Geometry check sheet. Reference: drawing and pictorial views, mm from the part's lowest x, y, z. Give positions to 0.01 mm unless a question says otherwise; leave off trailing zeros. Order: outer loops, then holes, each group sorted by start corner. A loop starts at its lowest first (then second) coordinate and runs counter-clockwise, first axis right, second up.
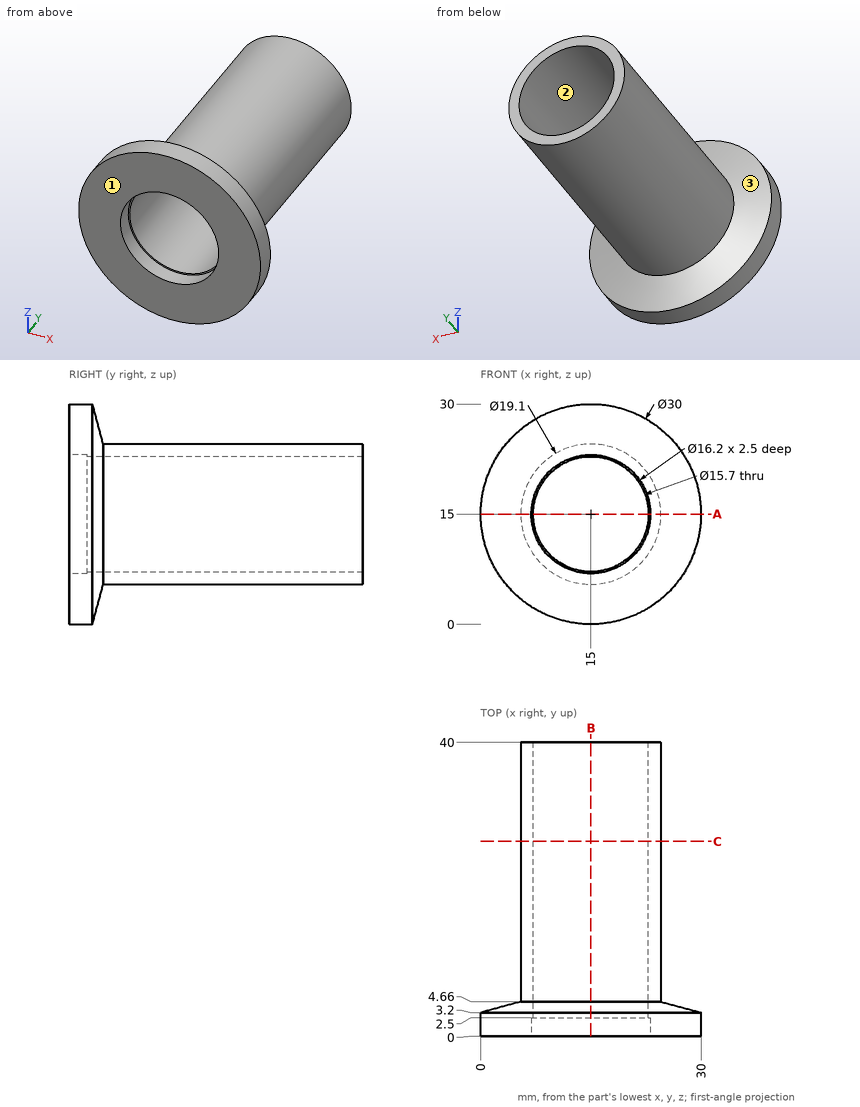
1) Draft check along Z on the marked faces 1, 2 and 3. Enter one of: +Z half, -Z half, draft (parallel to the pull), parting line (faces both ways), or undercut.
Recorded:
face 1: draft
face 2: undercut
face 3: parting line
2) Section check B-B, the plane x = 15. Record the cut outline in (y, z).
Recorded:
outline: (0, 0) - (3.2, 0) - (4.66, 5.45) - (40, 5.45) - (40, 7.15) - (2.5, 7.15) - (2.5, 6.9) - (0, 6.9) - close; (0, 23.1) - (2.5, 23.1) - (2.5, 22.85) - (40, 22.85) - (40, 24.55) - (4.66, 24.55) - (3.2, 30) - (0, 30) - close
3) Section check A-A, the plane z = 15. Record the cut outline in (x, y).
Recorded:
outline: (0, 0) - (6.9, 0) - (6.9, 2.5) - (7.15, 2.5) - (7.15, 40) - (5.45, 40) - (5.45, 4.66) - (0, 3.2) - close; (22.85, 2.5) - (23.1, 2.5) - (23.1, 0) - (30, 0) - (30, 3.2) - (24.55, 4.66) - (24.55, 40) - (22.85, 40) - close
4) Depth check by flat-ended pin: pin 1 Ø4 at (y, z) = (24.5, 25.5) entering from -X (1 decimal); pin 2 Ø4 at (x, z) = (10.5, 15.5) entering from -Y; pin 3 Ø1 at (y, z) = (29, 13) entering from -X; pin 4 Ø6 at (x, y) = (23.5, 17) entering from +Z. Enter the tip coordinate at first touch or a pass-through.
Recorded:
pin 1: stops at x = 10.6
pin 2: passes through
pin 3: stops at x = 5.57
pin 4: stops at z = 22.81
5) Material ranges on L1, parallel to X at y = 20.5, z = 15; L2, parallel to X at y = 1.55, z = 15; L3, parallel to Z at x = 13.75, y = 24, recorded low to high.
Recorded:
L1: x = 5.45 to 7.15, 22.85 to 24.55
L2: x = 0 to 6.9, 23.1 to 30
L3: z = 5.53 to 7.25, 22.75 to 24.47
6) Section check C-C, the plane y = 26.5. Record the cut outline in (x, z).
Recorded:
outline: circle Ø19.1 at (15, 15); hole circle Ø15.7 at (15, 15)
